Autodesk Inventor part; units mm, degrees
ref_plane "YZ Plane" through (0, 0, 0) normal (1, 0, 0) x (0, 1, 0)
ref_plane "XZ Plane" through (0, 0, 0) normal (0, 1, 0) x (-1, 0, 0)
ref_plane "XY Plane" through (0, 0, 0) normal (0, 0, 1) x (1, 0, 0)
sketch "Sketch1" plane through (0, 0, 0) normal (0, 0, 1) x (1, 0, 0)
  line L0 (0, 0) -> (3.175, 0)
  line L1 (3.175, 0) -> (3.175, 25.4)
  line L2 (3.175, 25.4) -> (0, 25.4)
  line L3 (0, 25.4) -> (0, 0)
  line L4 (0, 0) -> (25.4, 0)
  line L5 (25.4, 0) -> (25.4, 3.175)
  line L6 (25.4, 3.175) -> (0, 3.175)
  line L7 (0, 3.175) -> (0, 0)
  dimension "d0" = 3.175
  dimension "d1" = 25.4
  dimension "d2" = 25.4
  dimension "d3" = 3.175
extrude "Extrusion1" add sketch "Sketch1" along normal blind 508
sketch "Sketch2" plane through (3.175, 3.175, 0) normal (0, 1, 0) x (1, 0, 0)
  line L0 (-3.175, 0) -> (9.525, 0) construction
  line L1 (22.225, 0) -> (0, 0) construction
  line L2 (9.525, 0) -> (9.525, -12.7) construction
  circle A0 centre (9.525, -12.7) radius 2.5797
  line L3 (-3.175, -508) -> (22.225, -508) construction
  line L4 (9.525, -508) -> (9.525, -495.3) construction
  circle A1 centre (9.525, -495.3) radius 2.5826
  line L5 (-3.175, 0) -> (-3.175, -508) construction
  line L6 (-3.175, -254) -> (22.225, -254) construction
  line L7 (22.225, 0) -> (22.225, -508) construction
  line L8 (9.525, -495.3) -> (9.525, -254) construction
  circle A2 centre (9.525, -374.65) radius 2.5826
  circle A3 centre (9.525, -254) radius 2.5826
  line L9 (9.525, -254) -> (9.525, -12.7) construction
  circle A4 centre (9.525, -133.35) radius 2.5826
  dimension "d6" = 12.7
  dimension "d7" = 12.7
  dimension "d16" = 12.7
extrude "Extrusion3" cut sketch "Sketch2" against normal blind 533.4
properties part number "Bumper L"
Model file for the job. Use its own axes, mm. A direction names the side the tool comes from. Coordinates: 2 decimals unless noted, no trailing zeros. Order: outer loops, then holes, each group sorted by start corner. A loop starts at its lowest first (then second) coordinate and runs counter-clockwise, first axis right, second up. Notation, with made-up numbers: (84, 5.25) -> (131, 5.25) arc R18 ccw to (131, 26.25) -> close; hole circle Ø2 at (-26.5, 42.25). An arc over 180 degrees is marked (long way). Answer as a JSON object with one key per item and string values. Group by question number.
1) Flat gauge pins, fed straight in: pin 1 (4 mm diameter, centred on x = 20.5, z = 195.5, fed in from +Y) (3 decimals); pin 2 (6 mm diameter, centred on y = 12.5, z = 64.5, fed in from +X) (3 decimals). Where does each tip first touch, or does it go through?
2) Which spindle directions (+Z, -Z, +X, -X, +Y, -Y) get a long thin tool onto all of the face, cutting with end or side? Do faces 1 (the face through (3.175, 14, 250)), 2 (the face through (0, 13, 250)). Say none if no direction does.
3) Cut at B-B, the plane y = 9. Write the cut outline in (x, z) (3 decimals), then the cut area to 3 significant figures.
4) Cut at A-A, the plane z = 105. Write the cut outline in (x, y) (3 decimals), then the cut area to 3 significant figures.
5) Drill centre lines: L1, parallel to Z at x = 12.7, y = 1.5; L2, parallel to X at y = 1.85, z = 12.7; L3, parallel to Y at x = 10, z = 449.5 (3 decimals). Where is each one in solid material? Low to high.
Check values:
{
 "1": {"pin 1": "stops at y = 3.175", "pin 2": "stops at x = 3.175"},
 "2": {"face 1": "+Z, -Z, +X, +Y", "face 2": "+Z, -Z, -X, +Y, -Y"},
 "3": {"outline": "(0, 0) -> (3.175, 0) -> (3.175, 508) -> (0, 508) -> close", "area": "1,610 mm²"},
 "4": {"outline": "(0, 0) -> (25.4, 0) -> (25.4, 3.175) -> (3.175, 3.175) -> (3.175, 25.4) -> (0, 25.4) -> close", "area": "151 mm²"},
 "5": {"L1": "z = 0 to 10.12, 15.28 to 130.77, 135.93 to 251.42, 256.58 to 372.07, 377.23 to 492.72, 497.88 to 508", "L2": "x = 0 to 10.12, 15.28 to 25.4", "L3": "y = 0 to 3.175"}
}
